Here's how the part is built. I have some questions about the finished solid (model axes, mm). Face numbers are marked on the shaded views. A direction names the side the tool comes from. Give positions to 0.01 mm unless a question says otherwise; leave off trailing zeros. Write each loop counter-clockwise with the first axis right and the second up, starting at its lowest first coordinate (ties: lowest second). Pieces come first, ordered by that corner, then holes. Notation, with made-up numbers: (63, -29.75) -> (67, -29.75) arc R24 cw to (67, 2.25) -> close; hole circle Ø8 at (-0.75, 63.5). An arc over 180 degrees is marked (long way). Use one line per item in the form item = value.
```python
from build123d import *
from OCP.BRepFilletAPI import BRepFilletAPI_MakeChamfer

# Parameters (mm, degrees)
BOSS_EXTRUDE1_DEPTH                                  = 38.1
CBORE_FOR_3_8_BINDING_HEAD_MACHINE_SCREW_D           = 10.0838
CBORE_FOR_3_8_BINDING_HEAD_MACHINE_SCREW_CBORE_D     = 20.6756
CBORE_FOR_3_8_BINDING_HEAD_MACHINE_SCREW_CBORE_DEPTH = 3.175
FILLET1_R                                            = 2.54
FILLET2_R                                            = 6.35
CHAMFER1_SIZE                                        = 0.254
CHAMFER1_SIZE2                                       = 0.31888992
FILLET3_R                                            = 0.254
CHAMFER2_SIZE                                        = 0.254


with BuildPart() as part:
    # Sketch1 → Boss-Extrude1 (new body)
    with BuildSketch(Plane.XY):
        Polygon((0, 0), (44.45, 0), (44.45, -9.525), (0.5741924, -21.517102), (-7.6808076, -21.517102), (-7.6808076, -5.642102), (-38.1608076, -5.642102), (-38.1608076, 3.882898), (-14.0308076, 3.882898), (-6.35, 44.45), (0, 44.45), align=None)
    extrude(amount=BOSS_EXTRUDE1_DEPTH)

    # CBORE for 3/8 Binding Head Machine Screw1 (through all)
    with Locations(Plane(origin=(0, 3.882898, 0), x_dir=(1, 0, 0), z_dir=(0, 1, 0))):
        with Locations((-26.8578076, -19.05)):
            CounterBoreHole(CBORE_FOR_3_8_BINDING_HEAD_MACHINE_SCREW_D / 2, CBORE_FOR_3_8_BINDING_HEAD_MACHINE_SCREW_CBORE_D / 2, CBORE_FOR_3_8_BINDING_HEAD_MACHINE_SCREW_CBORE_DEPTH)

    # Fillet1
    fillet1_edges = [part.edges().sort_by_distance(p)[0] for p in [
        (-14.0308076, 3.882898, 19.05),
    ]]
    fillet(fillet1_edges, radius=FILLET1_R)

    # Fillet2
    fillet2_edges = [part.edges().sort_by_distance(p)[0] for p in [
        (0, 0, 19.05),
    ]]
    fillet(fillet2_edges, radius=FILLET2_R)

    # Chamfer1: one chamfer whose edges measure the first distance from different faces: ONE call of the kernel's chamfer builder (chamfer() names one face for all edges)
    chamfer1_edges_1 = [part.edges().sort_by_distance(p)[0] for p in [
        (25.4, 0, 0),
        (44.45, -4.7625, 0),
        (22.5120962, -15.521051, 0),
        (-3.5533076, -21.517102, 0),
        (-7.6808076, -13.579602, 0),
        (-9.994679571, 25.200189874, 38.1),
        (-22.9208076, -5.642102, 0),
        (-38.1608076, -0.879602, 0),
        (-9.994679571, 25.200189874, 0),
        (-3.175, 44.45, 0),
        (44.45, 0, 19.05),
        (-38.1608076, -5.642102, 19.05),
        (-38.1608076, 3.882898, 19.05),
        (0, 44.45, 19.05),
        (-38.1608076, -0.879602, 38.1),
        (-22.9208076, -5.642102, 38.1),
        (-7.6808076, -13.579602, 38.1),
        (-3.5533076, -21.517102, 38.1),
        (22.5120962, -15.521051, 38.1),
        (44.45, -4.7625, 38.1),
        (-27.147914139, 3.882898, 0),
        (-27.147914139, 3.882898, 38.1),
        (-14.514618931, 4.466907668, 0),
        (-14.514618931, 4.466907668, 38.1),
        (25.4, 0, 38.1),
        (0, 25.4, 0),
        (0, 25.4, 38.1),
        (1.859871939, 1.859871939, 0),
        (1.859871939, 1.859871939, 38.1),
        (-3.175, 44.45, 38.1),
    ]]
    chamfer1_edges_2 = [part.edges().sort_by_distance(p)[0] for p in [
        (-6.35, 44.45, 19.05),
    ]]
    chamfer1_side_2 = [part.faces().sort_by_distance(p)[0] for p in [
        (-3.175, 44.45, 19.05),
    ]]
    chamfer1 = BRepFilletAPI_MakeChamfer(part.part.solid().wrapped)
    for e in chamfer1_edges_1:
        chamfer1.Add(CHAMFER1_SIZE, e.wrapped)
    for e in chamfer1_edges_2:
        chamfer1.Add(CHAMFER1_SIZE, CHAMFER1_SIZE2, e.wrapped, chamfer1_side_2[0].wrapped)  # the first distance lies on this face
    add(Compound.cast(chamfer1.Shape()), mode=Mode.REPLACE)

    # Fillet3
    fillet3_edges = [part.edges().sort_by_distance(p)[0] for p in [
        (-37.1956076, 0.707898, 19.05),
    ]]
    fillet(fillet3_edges, radius=FILLET3_R)

    # Chamfer2
    chamfer2_edges = [part.edges().sort_by_distance(p)[0] for p in [
        (-21.8159076, -5.642102, 19.05),
    ]]
    chamfer(chamfer2_edges, length=CHAMFER2_SIZE)


solid = part.part
```
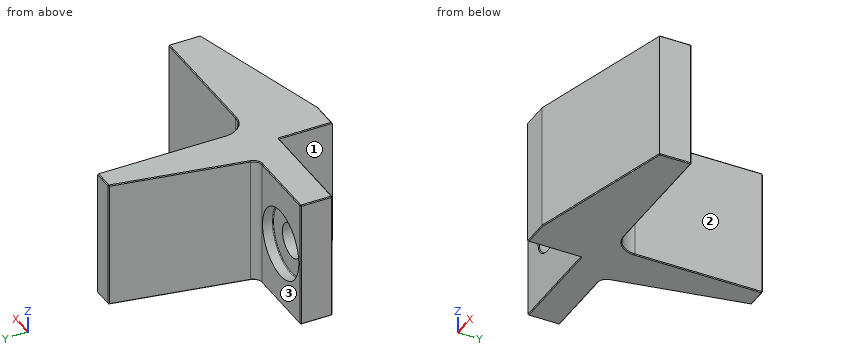
Q1. Which directions (+Z, -Z, +X, -X, +Y, -Y) give clear straight access to the entire face, cutting with the end or side of a thin tool? Please do the marked faces 1, 2 and 3.
Result set:
face_1 = +Z, -Z, -X, -Y
face_2 = +Z, -Z, +X, +Y
face_3 = +Z, -Z, -X, +Y
Q2. I want a section at D-D, the plane x = 23. Write out the boundary of the cut face in (y, z), and give its area (3 significant figures).
Result set:
outline = (-15.39, 0.25) -> (-15.12, 0) -> (-0.25, 0) -> (0, 0.25) -> (0, 37.85) -> (-0.25, 38.1) -> (-15.12, 38.1) -> (-15.39, 37.85) -> close
area = 586 mm2
Q3. I want a section at B-B, the plane y = -7. Write out the boundary of the cut face in (x, z).
Result set:
outline = (-7.68, 0.25) -> (-7.43, 0) -> (44.2, 0) -> (44.45, 0.25) -> (44.45, 37.85) -> (44.2, 38.1) -> (-7.43, 38.1) -> (-7.68, 37.85) -> close
Q4. Will these pins go through, and if not, where does the flat tip stop? pin 1 Ø9 at (x, z) = (-26.5, 24) entering from -Y; pin 2 Ø19 at (x, z) = (25, 27.5) entering from +Y; pin 3 Ø8 at (x, z) = (-26.86, 19.05) entering from -Y; pin 4 Ø1 at (y, z) = (23.5, 13.5) entering from -X.
Result set:
pin_1 = -5.64
pin_2 = 0
pin_3 = through
pin_4 = -10.41
Q5. If I drill on line 1 along X through (y, z) = (-1, 19); line 2 along X through (y, z) = (3, 19); line 3 along Y through (x, z) = (-19.5, 29.5), over which ranges is the centre line in solid material (lowest first)? Write a range as from..to.
Result set:
line_1 = -38.16..-31.9, -21.82..44.45
line_2 = -38.16..-37.2, -16.52..0.96
line_3 = -5.64..3.88
Q6. I want a section at C-C, the plane z = 32.5. Write out the boundary of the cut face in (x, y) (3 decimals), and give its area (3 significant figures).
Result set:
outline = (-38.161, -5.388) -> (-37.907, -5.642) -> (-7.681, -5.642) -> (-7.681, -21.517) -> (0.574, -21.517) -> (44.45, -9.525) -> (44.45, -0.254) -> (44.196, 0) -> (6.35, 0) arc R6.35 cw to (0, 6.35) -> (0, 44.196) -> (-0.254, 44.45) -> (-6.096, 44.45) -> (-6.409, 44.137) -> (-13.639, 5.95) arc R2.54 cw to (-16.135, 3.883) -> (-37.907, 3.883) -> (-38.161, 3.629) -> close
area = 1,600 mm2
